Build history of the part. All positions in model axes, mm. Give positions to 0.01 mm unless a question says otherwise; leave off trailing zeros. Write each loop counter-clockwise with the first axis right and the second up, starting at its lowest first coordinate (ties: lowest second). Pieces come first, ordered by that corner, then holes. Notation, with made-up numbers: M 48,-22 L 95,-22 A15 ccw 95,2 Z; hole C -24.5,54.25 d8. An arc over 180 degrees is marked long. Return JSON: item names as keys, results as strings. Group by question number.
Q1. Flat gauge pin, fed straight in: pin 1 Ø3 at (x, z) = (10, 160) entering from +Y. Where does the tip first touch, or does it go through?
Q2. Band-saw the part on D-D, the plane x = 3. Give the cut face in (y, z).
Q3. Pull direction Y, two halves, no side cores. Call faces 1 (the cylindrical face through (10.14, 10.631, 127.997)), 2 (the flat face through (10, 0, 94)), 3 (the cylindrical face through (10, 10, 178)), 4 (the cylindrical face through (10.14, 8.23, 61.13)): +Y half, -Y half, draft (parallel to the pull), parting line (faces both ways), or undercut.
Q4. Wall check: probe 1 along X at (y, z) = (10.75, 80); probe 2 along Y at (x, z) = (18.5, 130); probe 3 along Y at (x, z) = (4.25, 139). Give the ranges that are in metal, low to high.
Q5. Band-saw the part on C-C, the plane z = 80. Give the cut face in (x, y).
Q6. Band-saw the part on A-A, the plane x = 10. Count the separate pieces of the cut face and the enclosed holes in it, then the cut area to 3 significant figures.
from build123d import *

# Parameters (mm, degrees)
SKETCH_1_W               = 20
SKETCH_1_H               = 20
EXTRUDE_1_DEPTH          = 190
CUT_EXTRUDE_1_DEPTH      = 193.093727123
CUT_EXTRUDE_1_DEPTH_BACK = 193.093727123
SKETCH_2_R               = 2
SKETCH_2_R_2             = 2.5
SKETCH_3_R               = 2.1
CUT_EXTRUDE_2_DEPTH      = 193.093727123


with BuildPart() as part:
    # 草图1 → 凸台-拉伸1 (new body)
    with BuildSketch(Plane.XY):
        with Locations((10, 10)):
            Rectangle(SKETCH_1_W, SKETCH_1_H)
    extrude(amount=EXTRUDE_1_DEPTH)

    # 草图2 → 切除-拉伸1 (cut, two sides: drawn at the far end of the back side and taken through both)
    with BuildSketch(Plane(origin=(0, 20, 0), x_dir=(1, 0, 0), z_dir=(0, 1, 0)).offset(-CUT_EXTRUDE_1_DEPTH_BACK)):
        with Locations(Location((10, -180, 0), (0, 0, 270))):
            Circle(SKETCH_2_R)
        with Locations(Location((10, -160, 0), (0, 0, 270))):
            Circle(SKETCH_2_R)
        with Locations(Location((10, -110, 0), (0, 0, 270))):
            Circle(SKETCH_2_R_2)
        with Locations(Location((10, -10, 0), (0, 0, 90))):
            Circle(SKETCH_2_R)
        with Locations(Location((10, -30, 0), (0, 0, 90))):
            Circle(SKETCH_2_R)
        with Locations(Location((10, -80, 0), (0, 0, 90))):
            Circle(SKETCH_2_R_2)
    extrude(amount=CUT_EXTRUDE_1_DEPTH + CUT_EXTRUDE_1_DEPTH_BACK, mode=Mode.SUBTRACT)

    # 草图3 → 切除-拉伸2 (cut, through all)
    with BuildSketch(Plane(origin=(20, 0, 0), x_dir=(0, 0, -1), z_dir=(1, 0, 0))):
        with Locations((-140, 10)):
            Circle(SKETCH_3_R)
        with Locations((-130, 10)):
            Circle(SKETCH_3_R)
        with Locations((-150, 10)):
            Circle(SKETCH_3_R)
        with Locations(Location((-60, 10, 0), (0, 0, 180))):
            Circle(SKETCH_3_R)
        with Locations(Location((-50, 10, 0), (0, 0, 180))):
            Circle(SKETCH_3_R)
        with Locations(Location((-40, 10, 0), (0, 0, 180))):
            Circle(SKETCH_3_R)
    extrude(amount=-CUT_EXTRUDE_2_DEPTH, mode=Mode.SUBTRACT)


solid = part.part
From the geometry:
{
 "1": {"pin 1": "passes through"},
 "2": {"outline": "M 0,0 L 20,0 L 20,190 L 0,190 Z; hole C 10,40 d4.2; hole C 10,50 d4.2; hole C 10,60 d4.2; hole C 10,130 d4.2; hole C 10,140 d4.2; hole C 10,150 d4.2"},
 "3": {"face 1": "undercut", "face 2": "-Y half", "face 3": "draft", "face 4": "undercut"},
 "4": {"probe 1": "x = 0 to 7.5, 12.5 to 20", "probe 2": "y = 0 to 7.9, 12.1 to 20", "probe 3": "y = 0 to 8.15, 11.85 to 20"},
 "5": {"outline": "M 0,0 L 7.5,0 L 7.5,20 L 0,20 Z; M 12.5,0 L 20,0 L 20,20 L 12.5,20 Z"},
 "6": {"separate pieces": "7", "enclosed holes": "6", "area": "3,200 mm^2"}
}
